Model file for the job. Use its own axes, mm. Give positions to 0.01 mm unless a question says otherwise; leave off trailing zeros. Write each loop counter-clockwise with the first axis right and the second up, starting at its lowest first coordinate (ties: lowest second). Pieces come first, ordered by that corner, then holes.
```python
from build123d import *

# Parameters (mm, degrees)
SKETCH3_R           = 1.5
SKETCH3_W           = 229
SKETCH3_H           = 144
BOSS_EXTRUDE2_DEPTH = 2


with BuildPart() as part:
    # Sketch3 → Boss-Extrude2 (new body)
    with BuildSketch(Plane(origin=(0, 0, 0), x_dir=(1, 0, 0), z_dir=(0, 1, 0))):
        with BuildLine():
            Line((-127.15, 80.141387187), (-58.12279793, 80.141387187))
            ThreePointArc((-58.12279793, 80.141387187), (-52.819497071, 82.338086328), (-50.62279793, 87.641387187))
            Line((-50.62279793, 87.641387187), (-50.62279793, 91.641387187))
            ThreePointArc((-50.62279793, 91.641387187), (-46.961632695, 100.480221952), (-38.12279793, 104.141387187))
            Line((-38.12279793, 104.141387187), (36.87720207, 104.141387187))
            ThreePointArc((36.87720207, 104.141387187), (45.716036835, 100.480221952), (49.37720207, 91.641387187))
            Line((49.37720207, 91.641387187), (49.37720207, 87.641387187))
            ThreePointArc((49.37720207, 87.641387187), (51.573901211, 82.338086328), (56.87720207, 80.141387187))
            Line((56.87720207, 80.141387187), (127.15, 80.141387187))
            Line((127.15, 80.141387187), (127.15, -104.141387187))
            Line((127.15, -104.141387187), (-127.15, -104.141387187))
            Line((-127.15, -104.141387187), (-127.15, 80.141387187))
        make_face()
        with Locations((-124.667766953, 77.65915414)):
            Circle(SKETCH3_R, mode=Mode.SUBTRACT)
        with Locations((124.667766953, 77.65915414)):
            Circle(SKETCH3_R, mode=Mode.SUBTRACT)
        with Locations((124.667766953, -101.667766953)):
            Circle(SKETCH3_R, mode=Mode.SUBTRACT)
        with Locations((-124.667766953, -101.667766953)):
            Circle(SKETCH3_R, mode=Mode.SUBTRACT)
        with Locations((0, -12.008612813)):
            Rectangle(SKETCH3_W, SKETCH3_H, mode=Mode.SUBTRACT)
    extrude(amount=BOSS_EXTRUDE2_DEPTH)


solid = part.part
```
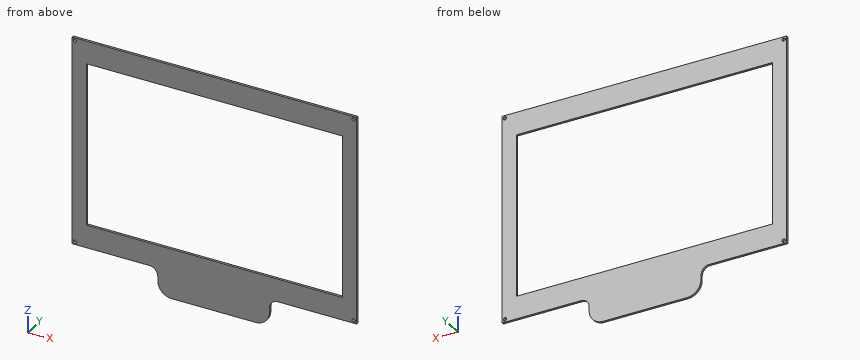
1. Pin check, flat tip, straight feed: P1, Ø0.6, axis at x = 102, y = 1.5, coming from the -Z side. Stop position of the tip, or through.
Calculated:
P1: stops at z = -80.14
2. Slice it at B-B, the plane z = -19.5. Write the cut outline in (x, y), and give its area (3 significant figures).
Calculated:
outline: (-127.15, 0) - (-114.5, 0) - (-114.5, 2) - (-127.15, 2) - close; (114.5, 0) - (127.15, 0) - (127.15, 2) - (114.5, 2) - close
area: 50.6 mm2
3. Slice it at C-C, the plane y = 0.75. Write the cut outline in (x, z), and give its area (3 significant figures).
Calculated:
outline: (-127.15, -80.14) - (-58.12, -80.14) arc R7.5 cw to (-50.62, -87.64) - (-50.62, -91.64) arc R12.5 ccw to (-38.12, -104.14) - (36.88, -104.14) arc R12.5 ccw to (49.38, -91.64) - (49.38, -87.64) arc R7.5 cw to (56.88, -80.14) - (127.15, -80.14) - (127.15, 104.14) - (-127.15, 104.14) - close; hole circle Ø3 at (-124.67, -77.66); hole circle Ø3 at (-124.67, 101.67); hole (-114.5, -59.99) - (114.5, -59.99) - (114.5, 84.01) - (-114.5, 84.01) - close; hole circle Ø3 at (124.67, -77.66); hole circle Ø3 at (124.67, 101.67)
area: 16,200 mm2
4. Slice it at A-A, the plane x = 5. Write the cut outline in (y, z).
Calculated:
outline: (0, -104.14) - (2, -104.14) - (2, -59.99) - (0, -59.99) - close; (0, 84.01) - (2, 84.01) - (2, 104.14) - (0, 104.14) - close
5. Probe probe 1 along X at (y, z) = (0.2, 18); probe 2 along Z at (x, y) = (-69, 0.5); probe 3 along X at (y, z) = (0.45, -78.5). List the from-to ranges inside material, lowest first.
Calculated:
probe 1: x = -127.15 to -114.5, 114.5 to 127.15
probe 2: z = -80.14 to -59.99, 84.01 to 104.14
probe 3: x = -127.15 to -125.91, -123.43 to 123.43, 125.91 to 127.15
